Geometry: see drawing. Coordinates: mm, zero at the bounding-box minimum. Give positions to 0.01 mm unless a question says otherwise; leave off trailing zeros. Loops run counter-clockwise (first coordinate to the right, second up) from the corner with the lowest first, then second, coordinate; pieces in that order, holes last. Notation, with made-up numbers: (74.25, -14.5) -> (112.25, -14.5) arc R20 cw to (112.25, -6.5) -> close; hole circle Ø1 at (-40, 68). An arc over 180 degrees is marked (long way). Return JSON: item names as keys, results as strings. Group by question number.
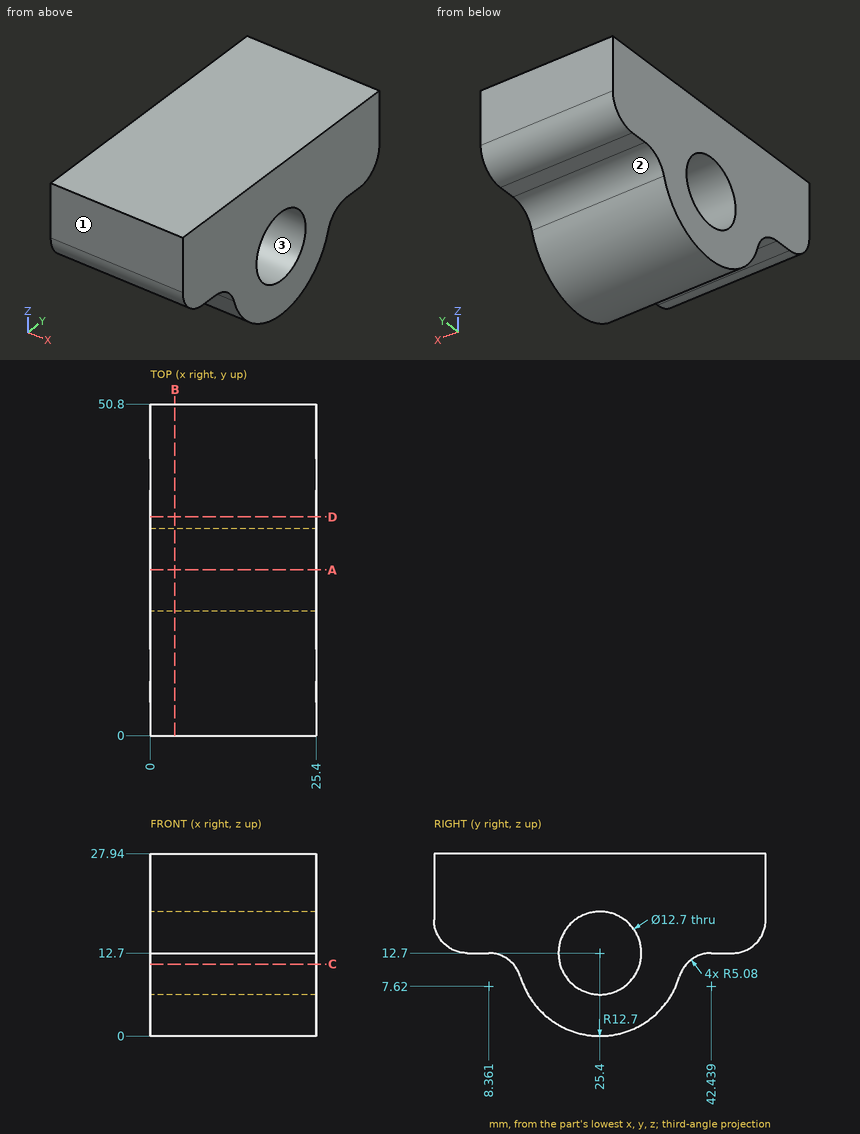
1) Contact query for flat-ended pins moving along their axis: P1, Ø3.5, axis at x = 8.5, y = 44.5, coming from the -Z side; P2, Ø7.5, axis at y = 25.4, z = 12.7, coming from the +X side; P3, Ø12, axis at x = 6.5, y = 33, coming from the -Z side; P4, Ø4, axis at x = 4, z = 15, coming from the +Y side. Output: stop coordinate, or through.
2) Cut plane B-B on x = 3.75. Return loops of the section in (y, z).
3) Cut plane D-D on y = 33.5. Return loops of the section in (x, z), then the cut area to 3 significant figures.
4) Cut plane C-C on z = 11. Return loops of the section in (x, y).
5) Mould query, pull axis Z, two halves, no side actions, for the marked faces 1, 2 and 3. Classes: released by +Z, released by -Z, zero draft, split by the parting line, or undercut.
6) Cut plane A-A on y = 25.4. Return loops of the section in (x, z), then the cut area to 3 significant figures.
7) Material intervals for line 1 (Z direction, x = 19.75, y = 21.5); line 2 (Y direction, x = 5, z = 9); line 3 (Y direction, x = 21.5, z = 16.5), sorted ascending.
Calculated:
{
 "1": {"P1": "z = 12.7", "P2": "through", "P3": "z = 0.1", "P4": "y = 50.74"},
 "2": {"outline": "(0, 17.78) arc R5.08 ccw to (5.08, 12.7) -> (8.36, 12.7) arc R5.08 cw to (13.23, 9.07) arc R12.7 ccw to (37.57, 9.07) arc R5.08 cw to (42.44, 12.7) -> (45.72, 12.7) arc R5.08 ccw to (50.8, 17.78) -> (50.8, 27.94) -> (0, 27.94) -> close; hole circle Ø12.7 at (25.4, 12.7)"},
 "3": {"outline": "(0, 2.92) -> (25.4, 2.92) -> (25.4, 27.94) -> (0, 27.94) -> close", "area": "636 mm2"},
 "4": {"outline": "(0, 12.15) -> (25.4, 12.15) -> (25.4, 19.28) -> (0, 19.28) -> close; (0, 31.52) -> (25.4, 31.52) -> (25.4, 38.65) -> (0, 38.65) -> close"},
 "5": {"face 1": "zero draft", "face 2": "released by -Z", "face 3": "undercut"},
 "6": {"outline": "(0, 0) -> (25.4, 0) -> (25.4, 6.35) -> (0, 6.35) -> close; (0, 19.05) -> (25.4, 19.05) -> (25.4, 27.94) -> (0, 27.94) -> close", "area": "387 mm2"},
 "7": {"line 1": "0.61 to 7.69, 17.71 to 27.94", "line 2": "13.25 to 20.24, 30.56 to 37.55", "line 3": "0.16 to 20.31, 30.49 to 50.64"}
}
